Part model, mm, in its own coordinate system. A direction names the side the tool comes from. Coordinates: 2 decimals unless noted, no trailing zeros. Order: outer loops, then holes, each group sorted by start corner. A loop starts at its lowest first (then second) coordinate and runs counter-clockwise, first axis right, second up. Notation, with made-up numbers: M 20.25,63 L 40.25,63 A30 ccw 40.25,93 Z; hole C 51.25,44 d2. An arc over 180 degrees is marked long. Write item = value, one per line. Start each with the question number.
from build123d import *

# Parameters (mm, degrees)
F0_W     = 238.125
F0_H     = 168.275
F1_DEPTH = 6.35
F3_DEPTH = 25.4
F4_DEPTH = 6.351
F6_DEPTH = 6.351
F7_R     = 5.08


with BuildPart() as f1:
    # F0 (on Top) → F1 (new body)
    with BuildSketch(Plane.XY):
        Rectangle(F0_W, F0_H)
    extrude(amount=F1_DEPTH)

    # F2 (on face) → F3 (cut)
    with BuildSketch(Plane.XY.offset(6.35)):
        Polygon((0, -22.479), (0, 67.437), (-44.958, 67.437), (-44.958, -67.437), (44.958, -67.437), (44.958, -22.479), align=None)
    extrude(amount=-F3_DEPTH, mode=Mode.SUBTRACT)

    # F2 (on face) → F4 (cut, through all)
    with BuildSketch(Plane.XY.offset(6.35)):
        Polygon((0, -22.479), (0, 67.437), (-44.958, 67.437), (-44.958, -67.437), (44.958, -67.437), (44.958, -22.479), align=None)
    extrude(amount=-F4_DEPTH, mode=Mode.SUBTRACT)

    # F5 (on face) → F6 (cut, through all)
    with BuildSketch(Plane.XY.offset(6.35)):
        with BuildLine():
            Line((1.27, -20.4216), (1.27, 67.9196))
            ThreePointArc((1.27, 67.9196), (1.039376, 68.476376), (0.4826, 68.707))
            Line((0.4826, 68.707), (-45.4406, 68.707))
            ThreePointArc((-45.4406, 68.707), (-45.997376, 68.476376), (-46.228, 67.9196))
            Line((-46.228, 67.9196), (-46.228, -67.9196))
            ThreePointArc((-46.228, -67.9196), (-45.997376, -68.476376), (-45.4406, -68.707))
            Line((-45.4406, -68.707), (45.4406, -68.707))
            ThreePointArc((45.4406, -68.707), (45.997376, -68.476376), (46.228, -67.9196))
            Line((46.228, -67.9196), (46.228, -21.9964))
            ThreePointArc((46.228, -21.9964), (45.997376, -21.439624), (45.4406, -21.209))
            Line((45.4406, -21.209), (2.0574, -21.209))
            ThreePointArc((2.0574, -21.209), (1.500624, -20.978376), (1.27, -20.4216))
        make_face()
    extrude(amount=-F6_DEPTH, mode=Mode.SUBTRACT)

    # F7
    f7_edges = [f1.edges().sort_by_distance(p)[0] for p in [
        (-119.0625, -84.1375, 3.175),
        (-119.0625, 84.1375, 3.175),
        (119.0625, -84.1375, 3.175),
        (119.0625, 84.1375, 3.175),
    ]]
    fillet(f7_edges, radius=F7_R)


solid = f1.part
Item 1: Cut at C-C, the plane z = 2.5. Write the cut outline in (x, y).
Item 2: Cut at B-B, the plane x = 34. Write the cut outline in (y, z), and give its area (3 significant figures).
Item 3: Pull direction X, two halves, no side cores. Call faces 1 (the cylindrical face through (117.535, 82.689, 3.219)), 2 (the cylindrical face through (-117.614, -82.61, 3.219)), 3 (the flat face through (24, -21.209, 3)): pulls with the +X half, pulls with the -X half, needs draft (parallel to the pull), parting line crosses it, or undercut.
Item 4: Wall check: line 1 along Y through (x, z) = (26.5, 1.25); line 2 along X through (y, z) = (4, 5.5); line 3 along X through (y, z) = (-27.5, 2.75). Give the ranges that are in metal, low to high. Write a range as [from, to].
Item 5: 3-axis set-ups, long thin cutter, end or side, ignore diameter. For faces 4 (the flat face through (-1, -68.707, 3)), 5 (the cylindrical face through (117.535, -82.689, 3.219)): which of +Z, -Z, +X, -X, +Y, -Y reach the whole face in a straight line?
Item 6: Cut at A-A, the plane y = 17.5. Write the cut outline in (x, z).
Filled sheet:
q1.outline = M -119.06,-79.06 A5.08 ccw -113.98,-84.14 L 113.98,-84.14 A5.08 ccw 119.06,-79.06 L 119.06,79.06 A5.08 ccw 113.98,84.14 L -113.98,84.14 A5.08 ccw -119.06,79.06 Z; hole M -46.23,-67.92 A0.79 ccw -45.44,-68.71 L 45.44,-68.71 A0.79 ccw 46.23,-67.92 L 46.23,-22 A0.79 ccw 45.44,-21.21 L 2.06,-21.21 A0.79 cw 1.27,-20.42 L 1.27,67.92 A0.79 ccw 0.48,68.71 L -45.44,68.71 A0.79 ccw -46.23,67.92 Z
q2.outline = M -84.14,0 L -68.71,0 L -68.71,6.35 L -84.14,6.35 Z; M -21.21,0 L 84.14,0 L 84.14,6.35 L -21.21,6.35 Z
q2.area = 767 mm2
q3.face_1 = pulls with the +X half
q3.face_2 = pulls with the -X half
q3.face_3 = undercut
q4.line_1 = [-84.14, -68.71], [-21.21, 84.14]
q4.line_2 = [-119.06, -46.23], [1.27, 119.06]
q4.line_3 = [-119.06, -46.23], [46.23, 119.06]
q5.face_4 = +Z, -Z
q5.face_5 = +Z, -Z, +X, -Y
q6.outline = M -119.06,0 L -46.23,0 L -46.23,6.35 L -119.06,6.35 Z; M 1.27,0 L 119.06,0 L 119.06,6.35 L 1.27,6.35 Z
